Build history of the part. All positions in model axes, mm. A direction names the side the tool comes from. Give positions to 0.01 mm unless a question says otherwise; leave off trailing zeros. Order: outer loops, then holes, each group sorted by start corner. A loop starts at its lowest first (then second) coordinate and runs counter-clockwise, first axis right, second up. Notation, with made-up numbers: (21, -23) -> (67, -23) arc R12 ccw to (67, -6) -> close; hole circle Ø3 at (34, 24.5). An arc over 180 degrees is marked (long way). One line per item, written item: value. Start each with the question number.
(1) Pin check, flat tip, straight feed: pin 1 (3 mm diameter, centred on x = -19, z = 25.5, fed in from +Y). Stop position of the tip, or through.
(2) Saw through at B-B on y = 17. Give the cut face in (x, z), plus the area to 3 significant figures.
(3) Which spindle directions (+Z, -Z, +X, -X, +Y, -Y) get a long thin tool onto all of the face, cutting with end or side? Do faces 5 (the cylindrical face through (1.182, 1.521, 12.221)), 6 (the flat face through (-2.318, 30, 35)), 7 (the flat face through (-26.318, 19, 10)). Say none if no direction does.
(4) Saw through at C-C on x = -24. Give the cut face in (y, z), plus the area to 3 significant figures.
(5) Two-plate mould, pull along Z, no slides. Class faces 1 (the flat face through (-7, 2, 8.754)), 2 (the flat face through (-8, 17, -17.246)), 3 (the cylindrical face through (3.8, 20, 35.3)), 4 (the flat face through (-7, 2, 13.754)): +Z half, -Z half, draft (parallel to the pull), parting line (faces both ways), or undercut.
(6) Probe line 1 (X direction, y = 11, z = 8); line 2 (Z direction, x = -17.5, y = 14); line 3 (Y direction, x = -21, z = 2). List the from-to ranges inside material, lowest first.
(7) Saw through at D-D on y = 32. Give the cut face in (x, z).
(8) Saw through at A-A on x = -5.5. Give the cut face in (y, z).
```python
from build123d import *

# Parameters (mm, degrees)
SCHIZZO1_W                   = 44
SCHIZZO1_H                   = 54
ESTRUSIONE_ESTRUSIONE1_DEPTH = 35
SVUOTA1_T                    = -3
TAGLIO_ESTRUSIONE1_DEPTH     = 57.871813174
TAGLIO_ESTRUSIONE2_REACH     = 72.714


with BuildPart() as part:
    # Schizzo1 → Estrusione-Estrusione1 (new body)
    with BuildSketch(Plane(origin=(0, 0, 0), x_dir=(1, 0, 0), z_dir=(0, 1, 0))):
        with Locations((-7.317535287, -9.754391008)):
            Rectangle(SCHIZZO1_W, SCHIZZO1_H)
    extrude(amount=ESTRUSIONE_ESTRUSIONE1_DEPTH)

    # Svuota1
    svuota1_openings = [part.faces().sort_by_distance(p)[0] for p in [
        (-7.317535287, 35, 9.754391008),
    ]]
    offset(amount=SVUOTA1_T, openings=svuota1_openings, kind=Kind.INTERSECTION)

    # Schizzo2 → Taglio-Estrusione1 (cut, through all)
    with BuildSketch(Plane(origin=(0, 3, 0), x_dir=(1, 0, 0), z_dir=(0, 1, 0))):
        with BuildLine():
            Line((-14.317535287, -0.754391008), (-0.317535287, -0.754391008))
            ThreePointArc((-0.317535287, -0.754391008), (1.182464713, -2.254391008), (-0.317535287, -3.754391008))
            Line((-0.317535287, -3.754391008), (-14.317535287, -3.754391008))
            ThreePointArc((-14.317535287, -3.754391008), (-15.817535287, -2.254391008), (-14.317535287, -0.754391008))
        make_face()
        with BuildLine():
            Line((-14.317535287, -5.754391008), (-0.317535287, -5.754391008))
            ThreePointArc((-0.317535287, -5.754391008), (1.182464713, -7.254391008), (-0.317535287, -8.754391008))
            Line((-0.317535287, -8.754391008), (-14.317535287, -8.754391008))
            ThreePointArc((-14.317535287, -8.754391008), (-15.817535287, -7.254391008), (-14.317535287, -5.754391008))
        make_face()
        with BuildLine():
            Line((-14.317535287, -10.754391008), (-0.317535287, -10.754391008))
            ThreePointArc((-0.317535287, -10.754391008), (1.182464713, -12.254391008), (-0.317535287, -13.754391008))
            Line((-0.317535287, -13.754391008), (-14.317535287, -13.754391008))
            ThreePointArc((-14.317535287, -13.754391008), (-15.817535287, -12.254391008), (-14.317535287, -10.754391008))
        make_face()
        with BuildLine():
            Line((-14.317535287, -15.754391008), (-0.317535287, -15.754391008))
            ThreePointArc((-0.317535287, -15.754391008), (1.182464713, -17.254391008), (-0.317535287, -18.754391008))
            Line((-0.317535287, -18.754391008), (-14.317535287, -18.754391008))
            ThreePointArc((-14.317535287, -18.754391008), (-15.817535287, -17.254391008), (-14.317535287, -15.754391008))
        make_face()
    extrude(amount=-TAGLIO_ESTRUSIONE1_DEPTH, mode=Mode.SUBTRACT)

    # Schizzo3 → Taglio-Estrusione2 (cut, up to next)
    with BuildSketch(Plane.XY.offset(36.754391008), mode=Mode.PRIVATE) as taglio_estrusione2_sk1:
        with BuildLine():
            Line((9.682464713, 35), (9.682464713, 26))
            ThreePointArc((9.682464713, 26), (3.682464713, 20), (-2.317535287, 26))
            Line((-2.317535287, 26), (-2.317535287, 35))
            Line((-2.317535287, 35), (9.682464713, 35))
        make_face()
    taglio_estrusione2_tool1 = extrude(taglio_estrusione2_sk1.sketch, amount=-TAGLIO_ESTRUSIONE2_REACH, mode=Mode.PRIVATE) & part.part
    add(taglio_estrusione2_tool1.solids().sort_by_distance((3.682465, 28.078412, 36.754391))[0], mode=Mode.SUBTRACT)


solid = part.part
```
Results below:
1. pin 1: stops at y = 3
2. outline: (-29.32, -17.25) -> (14.68, -17.25) -> (14.68, 36.75) -> (-29.32, 36.75) -> close; hole (-26.32, -14.25) -> (11.68, -14.25) -> (11.68, 33.75) -> (-26.32, 33.75) -> close
2. area: 552 mm²
3. face 5: +Y, -Y
3. face 6: +Z, +Y
3. face 7: +Y
4. outline: (0, -17.25) -> (35, -17.25) -> (35, -14.25) -> (3, -14.25) -> (3, 33.75) -> (35, 33.75) -> (35, 36.75) -> (0, 36.75) -> close
4. area: 354 mm²
5. face 1: undercut
5. face 2: -Z half
5. face 3: draft
5. face 4: undercut
6. line 1: x = -29.32 to -26.32, 11.68 to 14.68
6. line 2: z = -17.25 to -14.25, 33.75 to 36.75
6. line 3: y = 0 to 3
7. outline: (-29.32, -17.25) -> (14.68, -17.25) -> (14.68, 36.75) -> (9.68, 36.75) -> (9.68, 33.75) -> (11.68, 33.75) -> (11.68, -14.25) -> (-26.32, -14.25) -> (-26.32, 33.75) -> (-2.32, 33.75) -> (-2.32, 36.75) -> (-29.32, 36.75) -> close
8. outline: (0, -17.25) -> (35, -17.25) -> (35, -14.25) -> (3, -14.25) -> (3, 0.75) -> (0, 0.75) -> close; (0, 3.75) -> (3, 3.75) -> (3, 5.75) -> (0, 5.75) -> close; (0, 8.75) -> (3, 8.75) -> (3, 10.75) -> (0, 10.75) -> close; (0, 13.75) -> (3, 13.75) -> (3, 15.75) -> (0, 15.75) -> close; (0, 18.75) -> (3, 18.75) -> (3, 33.75) -> (35, 33.75) -> (35, 36.75) -> (0, 36.75) -> close
